Autodesk Inventor part; units mm, degrees
ref_plane "YZ Plane" through (0, 0, 0) normal (1, 0, 0) x (0, 1, 0)
ref_plane "XZ Plane" through (0, 0, 0) normal (0, 1, 0) x (-1, 0, 0)
ref_plane "XY Plane" through (0, 0, 0) normal (0, 0, 1) x (1, 0, 0)
sketch "Schizzo1" plane through (0, 0, 0) normal (0, 0, 1) x (1, 0, 0)
  line L0 (-10.5, 10) -> (10.5, 10)
  line L1 (10.5, 10) -> (10.5, -10)
  line L2 (10.5, -10) -> (-10.5, -10)
  line L3 (-10.5, -10) -> (-10.5, 10)
  line L4 (-10.5, 10) -> (10.5, -10) construction
  line L5 (10.5, 10) -> (-10.5, -10) construction
  line L6 (-7.3, 10) -> (-7.3, -10)
  line L7 (7.3, 10) -> (7.3, -10)
  line L8 (8.1, -10) -> (8.1, 10)
  line L9 (-8.1, -10) -> (-8.1, 10)
  point P0 (0, 0)
  point P1 (0, 0)
  dimension "d0" = 21
  dimension "d1" = 20
  dimension "d2" = 3.2
  dimension "d3" = 3.2
  dimension "d17" = 2.4
  dimension "d19" = 2.4
extrude "Estrusione4" add sketch "Schizzo1" along normal blind 2
extrude "Estrusione5" add sketch "Schizzo1" against normal blind 4 contours L0 L9 L2 L3 | L0 L6 L2 L9 | L0 L8 L2 L7 | L0 L1 L2 L8
extrude "Estrusione6" add sketch "Schizzo1" along normal blind 12 contours L0 L9 L2 L3 | L0 L1 L2 L8
fillet "Raccordo1" radius 1.2 2 edges at (8.1, 0, 2) (-8.1, 0, 2)
sketch "Schizzo3" plane through (-7.3, 10, 0) normal (0, 1, 0) x (1, 0, 0)
  line L0 (-3.2, 4) -> (-3.2, -12)
  line L1 (0, 4) -> (-3.2, 4)
  line L2 (-3.2, 0) -> (0, 4)
  line L3 (0, 4) -> (0, 0)
  line L4 (0, 0) -> (-3.2, 0)
  line L5 (14.6, 4) -> (17.8, 4)
  line L6 (14.6, 4) -> (17.8, 0)
  line L7 (17.8, 4) -> (17.8, -12)
  line L8 (14.6, 0) -> (14.6, 4)
  line L9 (14.6, 0) -> (17.8, 0)
  line L10 (-3.2, 0) -> (-3.2, 4)
  line L11 (0, 4) -> (-3.2, 4)
  line L12 (14.6, 4) -> (17.8, 4)
  line L13 (17.8, 0) -> (17.8, 4)
  point P0 (7.3, 0)
extrude "Estrusione7" cut sketch "Schizzo3" against normal blind 100 contours L1 L2 L0 | L5 L7 L6
fillet "Raccordo2" radius 2 2 edges at (-10.5, 0, 0) (10.5, 0, 0)
sketch "Schizzo4" plane through (-7.3, 10, 0) normal (0, 1, 0) x (1, 0, 0)
  line L0 (-3.2, -0.7016) -> (-3.2, -12)
  line L1 (-3.2, -1.9701) -> (-2, -12)
  line L2 (-0.8, -12) -> (-3.2, -12)
  line L3 (-2, -12) -> (-3.2, -12)
  line L4 (-3.2, -1.9701) -> (-3.2, -12)
  point P0 (7.3, 0)
extrude "Estrusione8" cut sketch "Schizzo4" against normal blind 100
mirror "Specchio1" about plane through (0, 0, 0) normal (1, 0, 0) of "Estrusione8"
properties part number "Sensore prossimale"
Could you check a few things on this model? Use its own coordinates, in mm. A direction names the side the tool comes from. Coordinates: 2 decimals unless noted, no trailing zeros. Order: outer loops, then holes, each group sorted by start corner. A loop starts at its lowest first (then second) coordinate and runs counter-clockwise, first axis right, second up. Notation, with made-up numbers: M 54,62 L 60,62 A19 ccw 60,75 Z; hole C 11,20.25 d7. An arc over 180 degrees is marked long. Use a Markdown table: item, result. Add a question column.
Q1. I want a section at B-B on y = 5.5. List the corners of the cut face in (x, z) for me, then the cut area to 3 significant figures.
Q2. If I drill on L1, parallel to Z at x = 1, y = -0.25; L2, parallel to X at y = -3.75, z = 9.5; L3, parallel to X at y = 9, z = 3.5, over which ranges is the centre line in solid material (lowest first)?
Q3. I want a section at D-D on x = 0.5. List the corners of the cut face in (y, z) for me, then the cut area to 3 significant figures.
Q4. I want a section at C-C on z = 3.5. List the corners of the cut face in (x, y) for me, then the cut area to 3 significant figures.
Q5. We'd pull the mould along X, two halves only. Please class faces 1 (the flat face through (9.89, 0.14, 7.06)), 2 (the flat face through (7.3, 0, -2)), 3 (the flat face through (0, -10, 1.6)): pulls with the +X half, pulls with the -X half, needs draft (parallel to the pull), parting line crosses it, or undercut.
Q6. I'm going to push flat-ended pins straight in: pin 1 (6 mm diameter, centred on x = -6, y = 7.5, fed in from -Z); pin 2 (1.2 mm diameter, centred on y = -3, z = -3, fed in from +X); pin 3 (9.5 mm diameter, centred on y = 4, z = 8.5, fed in from +X); pin 4 (2 mm diameter, centred on y = 0.5, z = -3, fed in from -X). Where does each tip first touch, or does it pass through?
Q7. I want a section at A-A on z = -2. List the corners of the cut face in (x, y) for me, then the cut area to 3 significant figures.
Q8. Which directions (+Z, -Z, +X, -X, +Y, -Y) give clear straight access to the entire face, cutting with the end or side of a thin tool? Please do faces 4 (the flat face through (8.1, 0, 8)), 5 (the flat face through (-7.3, 0, -2)), 6 (the flat face through (-10.5, 0, 1)).
Checked values:
| question | item | result |
|---|---|---|
| 1 | outline | M -10.5,0.7 A2 ccw -10.06,-0.55 L -7.3,-4 L -7.3,0 L 7.3,0 L 7.3,-4 L 10.06,-0.55 A2 ccw 10.5,0.7 L 10.5,1.97 L 9.3,12 L 8.1,12 L 8.1,3.2 A1.2 cw 6.9,2 L -6.9,2 A1.2 cw -8.1,3.2 L -8.1,12 L -9.3,12 L -10.5,1.97 Z |
| 1 | area | 91.3 mm² |
| 2 | L1 | 0 to 2 |
| 2 | L2 | -9.6 to -8.1, 8.1 to 9.6 |
| 2 | L3 | -10.32 to -8.1, 8.1 to 10.32 |
| 3 | outline | M -10,0 L 10,0 L 10,2 L -10,2 Z |
| 3 | area | 40.0 mm² |
| 4 | outline | M -10.32,-10 L -8.1,-10 L -8.1,10 L -10.32,10 Z; M 8.1,-10 L 10.32,-10 L 10.32,10 L 8.1,10 Z |
| 4 | area | 88.7 mm² |
| 5 | face 1 | pulls with the +X half |
| 5 | face 2 | undercut |
| 5 | face 3 | needs draft |
| 6 | pin 1 | z = -4 |
| 6 | pin 2 | x = 8.58 |
| 6 | pin 3 | x = 10.29 |
| 6 | pin 4 | x = -8.9 |
| 7 | outline | M -8.9,-10 L -7.3,-10 L -7.3,10 L -8.9,10 Z; M 7.3,-10 L 8.9,-10 L 8.9,10 L 7.3,10 Z |
| 7 | area | 64.0 mm² |
| 8 | face 4 | +Z, +Y, -Y |
| 8 | face 5 | -Z, +Y, -Y |
| 8 | face 6 | +Z, -Z, -X, +Y, -Y |
